```python
from build123d import *

# Parameters (mm, degrees)
SKETCH2_R                  = 4.5
BOSS_EXTRUDE1_DEPTH        = 10
BOSS_EXTRUDE5_DEPTH        = 22
BOSS_EXTRUDE5_DEPTH_BACK   = 48
BOSS_EXTRUDE6_DEPTH        = 48
F_16_0MM_DOWEL_HOLE1_D     = 16
F_16_0MM_DOWEL_HOLE1_DEPTH = 54
F_16_0MM_DOWEL_HOLE1_TIP   = 4.806884952


with BuildPart() as part:
    # Sketch2 → Boss-Extrude1 (new body)
    with BuildSketch(Plane(origin=(0, 0, 0), x_dir=(1, 0, 0), z_dir=(0, 1, 0))):
        with BuildLine():
            Line((11.936417534, 69.315868811), (49.936417534, 7.315868811))
            ThreePointArc((49.936417534, 7.315868811), (50.215198798, -6.840242563), (38, -14))
            Line((38, -14), (-38, -14))
            ThreePointArc((-38, -14), (-50.215198798, -6.840242563), (-49.936417534, 7.315868811))
            Line((-49.936417534, 7.315868811), (-11.936417534, 69.315868811))
            ThreePointArc((-11.936417534, 69.315868811), (0, 76), (11.936417534, 69.315868811))
        make_face()
        with Locations(Location((0, 62, 0), (0, 0, 270))):
            Circle(SKETCH2_R, mode=Mode.SUBTRACT)
        with Locations(Location((38, 0, 0), (0, 0, 270))):
            Circle(SKETCH2_R, mode=Mode.SUBTRACT)
        with Locations(Location((-38, 0, 0), (0, 0, 90))):
            Circle(SKETCH2_R, mode=Mode.SUBTRACT)
    extrude(amount=BOSS_EXTRUDE1_DEPTH)

    # Sketch3 → Boss-Extrude5 (add, two sides: drawn at the far end of the back side and taken through both)
    with BuildSketch(Plane.XY.offset(14).offset(-BOSS_EXTRUDE5_DEPTH_BACK)):
        with BuildLine():
            ThreePointArc((-8.732124598, 10), (-4.541475531, 8.137307921), (0, 7.5))
            Line((0, 7.5), (0, 10))
            Line((0, 10), (-8.732124598, 10))
        make_face()
        with BuildLine():
            Line((0, 10), (0, 7.5))
            ThreePointArc((0, 7.5), (4.541475531, 8.137307921), (8.732124598, 10))
            Line((8.732124598, 10), (0, 10))
        make_face()
        with BuildLine():
            Line((-8.732124598, 10), (0, 10))
            Line((0, 10), (0, 40.5))
            ThreePointArc((0, 40.5), (-11.66726189, 35.66726189), (-16.5, 24))
            ThreePointArc((-16.5, 24), (-14.427925282, 15.994691008), (-8.732124598, 10))
        make_face()
        with BuildLine():
            Line((0, 40.5), (0, 10))
            Line((0, 10), (8.732124598, 10))
            ThreePointArc((8.732124598, 10), (14.427925282, 15.994691008), (16.5, 24))
            ThreePointArc((16.5, 24), (11.66726189, 35.66726189), (0, 40.5))
        make_face()
    extrude(amount=BOSS_EXTRUDE5_DEPTH + BOSS_EXTRUDE5_DEPTH_BACK)

    # Sketch3_7 → Boss-Extrude6 (add)
    with BuildSketch(Plane.XY.offset(14)):
        with BuildLine():
            Line((16.5, 10), (16.5, 24))
            ThreePointArc((16.5, 24), (14.427925282, 15.994691008), (8.732124598, 10))
            Line((8.732124598, 10), (16.5, 10))
        make_face()
        with BuildLine():
            ThreePointArc((-8.732124598, 10), (-14.427925282, 15.994691008), (-16.5, 24))
            Line((-16.5, 24), (-16.5, 10))
            Line((-16.5, 10), (-8.732124598, 10))
        make_face()
    extrude(amount=-BOSS_EXTRUDE6_DEPTH)

    # 16.0mm Dowel Hole1
    with Locations(Plane.XY.offset(36)):
        with Locations((0, 24)):
            Hole(F_16_0MM_DOWEL_HOLE1_D / 2, depth=F_16_0MM_DOWEL_HOLE1_DEPTH)
            with Locations((0, 0, -(F_16_0MM_DOWEL_HOLE1_DEPTH + F_16_0MM_DOWEL_HOLE1_TIP / 2))):  # 118° drill point
                Cone(0, F_16_0MM_DOWEL_HOLE1_D / 2, F_16_0MM_DOWEL_HOLE1_TIP, mode=Mode.SUBTRACT)


solid = part.part
```
Part model, mm, in its own coordinate system. A direction names the side the tool comes from. Round coordinates to 2 decimals unless told otherwise and drop trailing zeros. Write each loop counter-clockwise with the first axis right and the second up, starting at its lowest first coordinate (ties: lowest second). Pieces come first, ordered by that corner, then holes. Notation, with made-up numbers: M -18,-29 L -5,-29 A25 ccw -5,-9 Z; hole C 5.5,66 d8. An arc over 180 degrees is marked long. One line per question, with ' | ' between items.
(1) Saw through at A-A on z = 0. Write the cut outline in (x, y), then the cut area to 3 significant figures.
Answer key:
outline: M -52,0 L -42.5,0 L -42.5,10 L -52,10 Z; M -33.5,0 L 33.5,0 L 33.5,10 L 16.5,10 L 16.5,24 A16.5 ccw -16.5,24 L -16.5,10 L -33.5,10 Z; M 42.5,0 L 52,0 L 52,10 L 42.5,10 Z; hole C 0,24 d16 | area: 1,550 mm^2
(2) Pin check, flat tips, straight feed: pin 1 (10 mm diameter, centred on x = -17, z = -20.5, fed in from +Y); pin 2 (2 mm diameter, centred on y = 29.5, z = 24.5, fed in from -X); pin 3 (18.5 mm diameter, centred on x = 0, y = 24, fed in from -Z); pin 4 (10 mm diameter, centred on x = -33.5, z = -17.5, fed in from -Y). Stop position of each tip, or through.
Answer key:
pin 1: stops at y = 35.32 | pin 2: stops at x = -15.87 | pin 3: stops at z = -34 | pin 4: stops at y = 0
(3) Saw through at D-D on y = 13. Write the cut outline in (x, z), then the cut area to 3 significant figures.
Answer key:
outline: M -16.5,-34 L 16.5,-34 L 16.5,14 L 12.3,14 L 12.3,36 L -12.3,36 L -12.3,14 L -16.5,14 Z | area: 2,130 mm^2
(4) 3-axis set-ups, long thin cutter, end or side, ignore diameter. For faces 4 (the face through (30.7, 4.9, -38.7)), 5 (the face through (0, 25, -34)), 6 (the face through (1, 10, -42)), 7 (the face through (16.5, 17, -10)), 8 (the face through (-16.5, 17, -10)): which of +Z, -Z, +X, -X, +Y, -Y reach the whole face in a straight line?
Answer key:
face 4: -Z, +X, +Y, -Y | face 5: -Z, +X, -X, +Y | face 6: -Z, +Y | face 7: +Z, -Z, +X, +Y | face 8: +Z, -Z, -X, +Y
(5) Two-plate mould, pull along Z, no slides. Class faces 1 (the face through (1.041, 31.932, 8.622)), 2 (the face through (-50.112, 4.93, 7.021)), 3 (the face through (-33.61, 4.93, 0.98)): released by +Z, released by -Z, zero draft, split by the parting line, or undercut.
Answer key:
face 1: zero draft | face 2: split by the parting line | face 3: undercut
(6) Probe line 1 along X through (y, z) = (4, 0); line 2 along Z through (x, y) = (-0.5, 9.5); line 3 along Y through (x, z) = (45.5, 8). List the from-to ranges inside material, lowest first.
Answer key:
line 1: x = -52 to -42.5, -33.5 to 33.5, 42.5 to 52 | line 2: z = -75.99 to -66.47, -57.53 to 36 | line 3: y = 0 to 10
(7) Saw through at B-B on x = -39.5. Write the cut outline in (y, z).
Answer key:
outline: M 0,-24.34 L 10,-24.34 L 10,-4.24 L 0,-4.24 Z; M 0,4.24 L 10,4.24 L 10,13.92 L 0,13.92 Z
(8) Saw through at C-C on z = -62. Write the cut outline in (x, y), then the cut area to 3 significant figures.
Answer key:
outline: M -16.42,0 L -4.5,0 L -4.5,10 L -16.42,10 Z; M 4.5,0 L 16.42,0 L 16.42,10 L 4.5,10 Z | area: 238 mm^2
